from build123d import *

# Parameters (mm, degrees)
SKETCH3_R            = 27.94
BOSS_EXTRUDE2_DEPTH  = 122.46
SKETCH5_R            = 3.175
CUT_EXTRUDE1_DEPTH   = 129.676877488
SKETCH4_W            = 14
SKETCH4_H            = 6
SHELL1_START         = 3
SHELL1_OUTLINE_R     = 10.94
SHELL1_OUTLINE_R_2   = 6.175
SHELL1_DEPTH         = 116.46
SHELL1_2_OUTLINE_R   = 24.94
SHELL1_2_OUTLINE_R_2 = 10.94
SHELL1_2_DEPTH       = 10.72
SHELL1_START_2       = 109.72
SHELL1_3_OUTLINE_R   = 24.94
SHELL1_3_OUTLINE_R_2 = 10.94
SHELL1_3_DEPTH       = 9.74
SHELL1_START_3       = 25.72
SHELL1_4_OUTLINE_R   = 24.94
SHELL1_4_OUTLINE_R_2 = 10.94
SHELL1_4_DEPTH       = 9
SHELL1_START_4       = 46.72
SHELL1_5_OUTLINE_R   = 24.94
SHELL1_5_OUTLINE_R_2 = 10.94
SHELL1_5_DEPTH       = 9
SHELL1_START_5       = 67.72
SHELL1_6_OUTLINE_R   = 24.94
SHELL1_6_OUTLINE_R_2 = 10.94
SHELL1_6_DEPTH       = 9
SHELL1_START_6       = 88.72
SHELL1_7_OUTLINE_R   = 24.94
SHELL1_7_OUTLINE_R_2 = 10.94
SHELL1_7_DEPTH       = 9
BOSS_EXTRUDE3_REACH  = 130.677
SKETCH13_W           = 16.483162312
SKETCH13_H           = 6
CUT_EXTRUDE3_DEPTH   = 123
BOSS_EXTRUDE4_DEPTH  = 122.46


# Read off the part's stored shape, not the designer's step: Shell1
with BuildPart() as part:
    # Sketch3 → Boss-Extrude2 (new body)
    with BuildSketch(Plane.XY):
        Circle(SKETCH3_R)
    extrude(amount=BOSS_EXTRUDE2_DEPTH)

    # Sketch5 → Cut-Extrude1 (cut, through all)
    with BuildSketch(Plane.XY.offset(122.46)):
        Circle(SKETCH5_R)
    extrude(amount=-CUT_EXTRUDE1_DEPTH, mode=Mode.SUBTRACT)

    # Sketch4 → Cut-Revolve1 (revolve, cut)
    with BuildSketch(Plane(origin=(0, 0, 0), x_dir=(1, 0, 0), z_dir=(0, 1, 0)), mode=Mode.PRIVATE) as cut_revolve1_sk:
        with Locations((-20.94, -103.72)):
            Rectangle(SKETCH4_W, SKETCH4_H)
        with Locations((-20.94, -82.72)):
            Rectangle(SKETCH4_W, SKETCH4_H)
        with Locations((-20.94, -61.72)):
            Rectangle(SKETCH4_W, SKETCH4_H)
        with Locations((-20.94, -40.72)):
            Rectangle(SKETCH4_W, SKETCH4_H)
        with Locations((-20.94, -19.72)):
            Rectangle(SKETCH4_W, SKETCH4_H)
    revolve(cut_revolve1_sk.sketch.rotate(Axis((0, 0, 122.46), (0, 0, -1)), 180), axis=Axis((0, 0, 122.46), (0, 0, -1)), mode=Mode.SUBTRACT)

    # Shell1 outline → Shell1 (cut)
    with BuildSketch(Plane.XY.offset(SHELL1_START)):
        Circle(SHELL1_OUTLINE_R)
        Circle(SHELL1_OUTLINE_R_2, mode=Mode.SUBTRACT)
    extrude(amount=SHELL1_DEPTH, mode=Mode.SUBTRACT)

    # Shell1 2 outline → Shell1 2 (cut)
    with BuildSketch(Plane.XY.offset(SHELL1_START)):
        Circle(SHELL1_2_OUTLINE_R)
        Circle(SHELL1_2_OUTLINE_R_2, mode=Mode.SUBTRACT)
    extrude(amount=SHELL1_2_DEPTH, mode=Mode.SUBTRACT)

    # Shell1 3 outline → Shell1 3 (cut)
    with BuildSketch(Plane.XY.offset(SHELL1_START_2)):
        Circle(SHELL1_3_OUTLINE_R)
        Circle(SHELL1_3_OUTLINE_R_2, mode=Mode.SUBTRACT)
    extrude(amount=SHELL1_3_DEPTH, mode=Mode.SUBTRACT)

    # Shell1 4 outline → Shell1 4 (cut)
    with BuildSketch(Plane.XY.offset(SHELL1_START_3)):
        Circle(SHELL1_4_OUTLINE_R)
        Circle(SHELL1_4_OUTLINE_R_2, mode=Mode.SUBTRACT)
    extrude(amount=SHELL1_4_DEPTH, mode=Mode.SUBTRACT)

    # Shell1 5 outline → Shell1 5 (cut)
    with BuildSketch(Plane.XY.offset(SHELL1_START_4)):
        Circle(SHELL1_5_OUTLINE_R)
        Circle(SHELL1_5_OUTLINE_R_2, mode=Mode.SUBTRACT)
    extrude(amount=SHELL1_5_DEPTH, mode=Mode.SUBTRACT)

    # Shell1 6 outline → Shell1 6 (cut)
    with BuildSketch(Plane.XY.offset(SHELL1_START_5)):
        Circle(SHELL1_6_OUTLINE_R)
        Circle(SHELL1_6_OUTLINE_R_2, mode=Mode.SUBTRACT)
    extrude(amount=SHELL1_6_DEPTH, mode=Mode.SUBTRACT)

    # Shell1 7 outline → Shell1 7 (cut)
    with BuildSketch(Plane.XY.offset(SHELL1_START_6)):
        Circle(SHELL1_7_OUTLINE_R)
        Circle(SHELL1_7_OUTLINE_R_2, mode=Mode.SUBTRACT)
    extrude(amount=SHELL1_7_DEPTH, mode=Mode.SUBTRACT)

    # Boss-Extrude3: up to this face of the body (flat: up to its plane)
    boss_extrude3_end = Plane(part.part.faces().sort_by_distance((-27.149737461, 0, 122.46))[0])
    # Sketch10 → Boss-Extrude3 (add, up to the picked face)
    with BuildSketch(Plane(origin=(0, 0, 0), x_dir=(-1, 0, 0), z_dir=(0, 0, -1)), mode=Mode.PRIVATE) as boss_extrude3_sk1:
        with BuildLine():
            Line((-1, 27.922098775), (-1, 3.01340754))
            ThreePointArc((-1, 3.01340754), (0, 3.175), (1, 3.01340754))
            Line((1, 3.01340754), (1, 27.922098775))
            ThreePointArc((1, 27.922098775), (0, 27.94), (-1, 27.922098775))
        make_face()
    boss_extrude3_tool1 = split(extrude(boss_extrude3_sk1.sketch, amount=-BOSS_EXTRUDE3_REACH, mode=Mode.PRIVATE), bisect_by=boss_extrude3_end, keep=Keep.BOTH, mode=Mode.PRIVATE)
    # Sketch10 → Boss-Extrude3 (add, up to the picked face)
    with BuildSketch(Plane(origin=(0, 0, 0), x_dir=(-1, 0, 0), z_dir=(0, 0, -1)), mode=Mode.PRIVATE) as boss_extrude3_sk2:
        with BuildLine():
            Line((3.01340754, 1), (27.922098775, 1))
            ThreePointArc((27.922098775, 1), (27.94, 0), (27.922098775, -1))
            Line((27.922098775, -1), (3.01340754, -1))
            ThreePointArc((3.01340754, -1), (3.175, 0), (3.01340754, 1))
        make_face()
    boss_extrude3_tool2 = split(extrude(boss_extrude3_sk2.sketch, amount=-BOSS_EXTRUDE3_REACH, mode=Mode.PRIVATE), bisect_by=boss_extrude3_end, keep=Keep.BOTH, mode=Mode.PRIVATE)
    # Sketch10 → Boss-Extrude3 (add, up to the picked face)
    with BuildSketch(Plane(origin=(0, 0, 0), x_dir=(-1, 0, 0), z_dir=(0, 0, -1)), mode=Mode.PRIVATE) as boss_extrude3_sk3:
        with BuildLine():
            Line((-1, -3.01340754), (-1, -27.922098775))
            ThreePointArc((-1, -27.922098775), (0, -27.94), (1, -27.922098775))
            Line((1, -27.922098775), (1, -3.01340754))
            ThreePointArc((1, -3.01340754), (0, -3.175), (-1, -3.01340754))
        make_face()
    boss_extrude3_tool3 = split(extrude(boss_extrude3_sk3.sketch, amount=-BOSS_EXTRUDE3_REACH, mode=Mode.PRIVATE), bisect_by=boss_extrude3_end, keep=Keep.BOTH, mode=Mode.PRIVATE)
    # Sketch10 → Boss-Extrude3 (add, up to the picked face)
    with BuildSketch(Plane(origin=(0, 0, 0), x_dir=(-1, 0, 0), z_dir=(0, 0, -1)), mode=Mode.PRIVATE) as boss_extrude3_sk4:
        with BuildLine():
            Line((-27.922098775, -1), (-3.01340754, -1))
            ThreePointArc((-3.01340754, -1), (-3.175, 0), (-3.01340754, 1))
            Line((-3.01340754, 1), (-27.922098775, 1))
            ThreePointArc((-27.922098775, 1), (-27.94, 0), (-27.922098775, -1))
        make_face()
    boss_extrude3_tool4 = split(extrude(boss_extrude3_sk4.sketch, amount=-BOSS_EXTRUDE3_REACH, mode=Mode.PRIVATE), bisect_by=boss_extrude3_end, keep=Keep.BOTH, mode=Mode.PRIVATE)
    add(boss_extrude3_tool1.solids().sort_by(Axis((0, 15.527819, 0), (0, 0, 1)))[0])
    add(boss_extrude3_tool2.solids().sort_by(Axis((-15.527819, 0, 0), (0, 0, 1)))[0])
    add(boss_extrude3_tool3.solids().sort_by(Axis((0, -15.527819, 0), (0, 0, 1)))[0])
    add(boss_extrude3_tool4.solids().sort_by(Axis((15.527819, 0, 0), (0, 0, 1)))[0])

    # Sketch13 → Cut-Revolve2 (revolve, cut)
    with BuildSketch(Plane(origin=(0, 0, 0), x_dir=(1, 0, 0), z_dir=(0, 1, 0)), mode=Mode.PRIVATE) as cut_revolve2_sk:
        with Locations((-22.145666886, -40.72)):
            Rectangle(SKETCH13_W, SKETCH13_H)
        with Locations((-22.145666886, -19.72)):
            Rectangle(SKETCH13_W, SKETCH13_H)
        with Locations((-22.145666886, -61.72)):
            Rectangle(SKETCH13_W, SKETCH13_H)
        with Locations((-22.145666886, -82.72)):
            Rectangle(SKETCH13_W, SKETCH13_H)
        with Locations((-22.145666886, -103.72)):
            Rectangle(SKETCH13_W, SKETCH13_H)
    revolve(cut_revolve2_sk.sketch.rotate(Axis((0, 0, 121.588746248), (0, 0, -1)), 180), axis=Axis((0, 0, 121.588746248), (0, 0, -1)), mode=Mode.SUBTRACT)

    # Sketch16 → Cut-Extrude3 (cut)
    with BuildSketch(Plane(origin=(0, 0, 0), x_dir=(-1, 0, 0), z_dir=(0, 0, -1))):
        with BuildLine():
            Line((-27.923120749, -0.971044624), (-6.098171639, -0.971044624))
            ThreePointArc((-6.098171639, -0.971044624), (-0.014665674, -6.174982584), (6.093490379, -1))
            Line((6.093490379, -1), (27.922098775, -1))
            ThreePointArc((27.922098775, -1), (-0.014486703, -27.939996244), (-27.923120749, -0.971044624))
        make_face()
    extrude(amount=-CUT_EXTRUDE3_DEPTH, mode=Mode.SUBTRACT)

    # Sketch17 → Boss-Extrude4 (add)
    with BuildSketch(Plane(origin=(0, 0, 0), x_dir=(-1, 0, 0), z_dir=(0, 0, -1))):
        with BuildLine():
            Line((-6.098171639, -0.971044624), (-7.108987082, -0.971044624))
            ThreePointArc((-7.108987082, -0.971044624), (-0.014616223, -7.174985113), (7.104971851, -1))
            Line((7.104971851, -1), (6.093490379, -1))
            ThreePointArc((6.093490379, -1), (-0.014665674, -6.174982584), (-6.098171639, -0.971044624))
        make_face()
    extrude(amount=-BOSS_EXTRUDE4_DEPTH)


solid = part.part
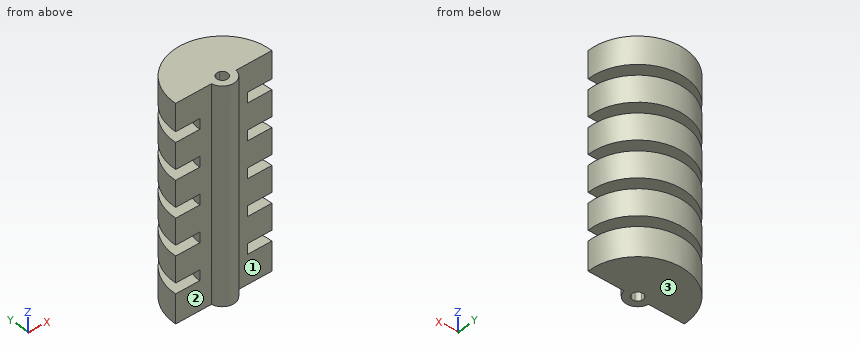
Design review of the part built by this model. Coordinates are the model's own, in mm. Face numbers are marked on the shaded views. A direction names the side the tool comes from. Give positions to 0.01 mm unless a question says otherwise; leave off trailing zeros. Return JSON: item names as keys, results as strings. Group by question number.
Item 1: Take a section at A-A (z = 32.5). Count the separate pieces of the cut face and the enclosed holes in it, plus the area to 3 significant figures.
Item 2: Clearance check with flat-ended pins moving along their axes: pin 1 Ø1.5 at (y, z) = (24, 55.5) entering from +X; pin 2 Ø2 at (y, z) = (3.5, 68) entering from +X; pin 3 Ø4 at (y, z) = (6.5, 12.5) entering from -X. State where each tip first meets the part, or that it passes through.
Item 3: Wall thickness on line 1 along Z through (x, y) = (-23, 13); line 2 along Z through (x, y) = (-4.5, 8); line 3 along X through (y, z) = (8.5, 93): over which ranges is each line inside the solid? List them lowest first.
Item 4: Tool access review of the marked faces 1, 2 and 3: name each direction out of +Z, -Z, +X, -X, +Y, -Y from which nothing blocks a thin tool from reaching the whole face with its end or side.
Return value:
{
 "1": {"separate pieces": "1", "enclosed holes": "3", "area": "474 mm2"},
 "2": {"pin 1": "stops at x = 15.49", "pin 2": "stops at x = 27.83", "pin 3": "stops at x = -27.58"},
 "3": {"line 1": "z = 0 to 16.72, 22.72 to 37.72, 43.72 to 58.72, 64.72 to 79.72, 85.72 to 100.72, 106.72 to 122.46", "line 2": "z = 0 to 3, 119.46 to 122.46", "line 3": "x = -26.62 to -23.45, -1 to 1, 23.45 to 26.62"},
 "4": {"face 1": "+Z, -Z, +X, -Y", "face 2": "+Z, -Z, -X, -Y", "face 3": "-Z, +X, -X, +Y, -Y"}
}
